```python
from build123d import *

# Parameters (mm, degrees)
SKETCH_1_W          = 151
SKETCH_1_H          = 46.5
EXTRUDE_1_DEPTH     = 14.6
SKETCH_5_W          = 4
SKETCH_5_H          = 13.25
EXTRUDE_5_DEPTH     = 3
SKETCH1_W           = 147
SKETCH1_H           = 43
CUT_EXTRUDE1_DEPTH  = 11
SKETCH2_W           = 14.914313068
SKETCH2_H           = 1.75
CUT_EXTRUDE2_DEPTH  = 11
SKETCH_8_W          = 28.4
SKETCH_8_H          = 46.5
BOSS_EXTRUDE1_DEPTH = 2


with BuildPart() as part:
    # 草图1 → 凸台-拉伸1 (new body)
    with BuildSketch(Plane(origin=(0, 0, 0), x_dir=(1, 0, 0), z_dir=(0, 1, 0))):
        Rectangle(SKETCH_1_W, SKETCH_1_H)
    extrude(amount=EXTRUDE_1_DEPTH)

    # 草图5 → 凸台-拉伸5 (add)
    with BuildSketch(Plane(origin=(0, 0, 0), x_dir=(-1, 0, 0), z_dir=(0, -1, 0))):
        with Locations((-12.2, -16.625)):
            Rectangle(SKETCH_5_W, SKETCH_5_H)
        with Locations((12.2, -16.625)):
            Rectangle(SKETCH_5_W, SKETCH_5_H)
        with Locations((-12.2, 16.625)):
            Rectangle(SKETCH_5_W, SKETCH_5_H)
        with Locations((12.2, 16.625)):
            Rectangle(SKETCH_5_W, SKETCH_5_H)
    extrude(amount=EXTRUDE_5_DEPTH)

    # Sketch1 → Cut-Extrude1 (cut)
    with BuildSketch(Plane(origin=(0, 14.6, 0), x_dir=(1, 0, 0), z_dir=(0, 1, 0))):
        Rectangle(SKETCH1_W, SKETCH1_H)
    extrude(amount=-CUT_EXTRUDE1_DEPTH, mode=Mode.SUBTRACT)

    # Sketch2 → Cut-Extrude2 (cut)
    with BuildSketch(Plane(origin=(0, 14.6, 0), x_dir=(1, 0, 0), z_dir=(0, 1, 0))):
        with Locations((-48.957156534, 22.375)):
            Rectangle(SKETCH2_W, SKETCH2_H)
    extrude(amount=-CUT_EXTRUDE2_DEPTH, mode=Mode.SUBTRACT)

    # 草图8 → Boss-Extrude1 (add)
    with BuildSketch(Plane(origin=(0, -3, 0), x_dir=(-1, 0, 0), z_dir=(0, -1, 0))):
        Rectangle(SKETCH_8_W, SKETCH_8_H)
    extrude(amount=BOSS_EXTRUDE1_DEPTH)


solid = part.part
```
Check sheet for the modelled part. Datum: model origin and axes. Units: mm. A direction names the side the tool comes from. Round coordinates to 2 decimals unless told otherwise and drop trailing zeros. Order: outer loops, then holes, each group sorted by start corner. A loop starts at its lowest first (then second) coordinate and runs counter-clockwise, first axis right, second up. Notation, with made-up numbers: (9, -3.5) -> (66, -3.5) arc R27 ccw to (66, 35.5) -> close; hole circle Ø6 at (11, 69). An arc over 180 degrees is marked (long way). Use CSV: the item, a comma, the result in double quotes.
(1) Cross-section at C-C (y = 11). Record the boundary of the cut face in (x, z), and give its area (3 significant figures).
Worked out:
outline,"(-75.5, -23.25) -> (-56.41, -23.25) -> (-56.41, -21.5) -> (-73.5, -21.5) -> (-73.5, 21.5) -> (73.5, 21.5) -> (73.5, -21.5) -> (-41.5, -21.5) -> (-41.5, -23.25) -> (75.5, -23.25) -> (75.5, 23.25) -> (-75.5, 23.25) -> close"
area,"674 mm²"
(2) Cross-section at D-D (z = -0.5). Record the boundary of the cut face in (x, y).
Worked out:
outline,"(-75.5, 0) -> (75.5, 0) -> (75.5, 14.6) -> (73.5, 14.6) -> (73.5, 3.6) -> (-73.5, 3.6) -> (-73.5, 14.6) -> (-75.5, 14.6) -> close; (-14.2, -5) -> (14.2, -5) -> (14.2, -3) -> (-14.2, -3) -> close"
(3) Tool access check on faces 5 (the face through (1, 7, 23.25)), 6 (the face through (-73.5, 9, 0)), 7 (the face through (12, -1, 10)), 8 (the face through (-10.2, -1, -17)). Record the directions out of +Z, -Z, +X, -X, +Y, -Y that give a thin tool (end or side, any length) a straight path to the whole face; none if there is none.
Worked out:
face 5,"+Z, +X, -X, +Y, -Y"
face 6,"+Y"
face 7,"+X, -X"
face 8,"+Z, -Z"
(4) Cross-section at A-A (z = 15.5). Record the boundary of the cut face in (x, y).
Worked out:
outline,"(-75.5, 0) -> (-14.2, 0) -> (-14.2, -5) -> (14.2, -5) -> (14.2, 0) -> (75.5, 0) -> (75.5, 14.6) -> (73.5, 14.6) -> (73.5, 3.6) -> (-73.5, 3.6) -> (-73.5, 14.6) -> (-75.5, 14.6) -> close; hole (-10.2, -3) -> (10.2, -3) -> (10.2, 0) -> (-10.2, 0) -> close"
(5) Material ranges on line 1 along Y through (x, z) = (-0.5, -19.5); line 2 along X through (y, z) = (13.25, 1.5); line 3 along Z through (x, y) = (-5.5, 11.5), recorded low to high. Write a range as from..to.
Worked out:
line 1,"-5..-3, 0..3.6"
line 2,"-75.5..-73.5, 73.5..75.5"
line 3,"-23.25..-21.5, 21.5..23.25"
(6) Depth check by flat-ended pin: pin 1 (14 mm diameter, centred on x = -3.5, z = -0.5, fed in from +Y); pin 2 (3.5 mm diameter, centred on y = -1.5, z = -18.5, fed in from -X); pin 3 (0.9 mm diameter, centred on y = -1.5, z = -17, fed in from +X); pin 4 (1 mm diameter, centred on x = 47.5, z = -2.5, fed in from -Y). Enter the tip coordinate at first touch or a pass-through.
Worked out:
pin 1,"y = 3.6"
pin 2,"x = -75.5"
pin 3,"x = 14.2"
pin 4,"y = 0"
(7) Draft check along X on faces 1 (the face through (0, -3, 0)), 2 (the face through (0, -5, 0)), 3 (the face through (75.5, 7, 0)), 4 (the face through (10.2, -1, 17)). Enter one of: pulls with the +X half, pulls with the -X half, needs draft (parallel to the pull), parting line crosses it, or undercut.
Worked out:
face 1,"undercut"
face 2,"needs draft"
face 3,"pulls with the +X half"
face 4,"undercut"
(8) Cross-section at B-B (x = 7.5). Record the boundary of the cut face in (y, z), and give its area (3 significant figures).
Worked out:
outline,"(-5, -23.25) -> (-3, -23.25) -> (-3, 23.25) -> (-5, 23.25) -> close; (0, -23.25) -> (14.6, -23.25) -> (14.6, -21.5) -> (3.6, -21.5) -> (3.6, 21.5) -> (14.6, 21.5) -> (14.6, 23.25) -> (0, 23.25) -> close"
area,"299 mm²"
